Source: CAD feature listing. Evaluate the final solid. Frame: model axes, mm. Face numbers are marked on the shaded views. A direction names the side the tool comes from. Round coordinates to 2 decimals unless told otherwise and drop trailing zeros. Loops run counter-clockwise (first coordinate to the right, second up) from the corner with the lowest first, then second, coordinate; pieces in that order, holes last.
Item 1: First-contact query: P1, Ø1.8, axis at x = -1.12, z = 1.56, coming from the -Y side. Flat tip, straight axial feed; report the tip coordinate or a pass-through.
Item 2: Section query C-C on x = 0.25. Return loops of the section in (y, z), then the cut area to 3 significant figures.
Item 3: Access query for the marked faces 4, 5 and 6. Directions: +Z, -Z, +X, -X, +Y, -Y. A direction counts if a zero-diameter tool reaches every point of the face in a straight line with its end or side. Return the directions, or none.
Item 4: Section query D-D on x = 5.75. Return loops of the section in (y, z), then the cut area to 3 significant figures.
Item 5: Pull-direction query (Z, two-part tool) for the marked faces 1, 2 and 3; classes: released by +Z, released by -Z, zero draft, split by the parting line, or undercut.
Item 6: Ray query, L1, parallel to X at y = 1.2, z = 1.5; L2, parallel to Z at x = -1.5, y = 1.25; L3, parallel to X at y = 1.75, z = -4.5. Return the intervals inside material, ascending.
Item 7: Section query A-A on z = 2.75. Return loops of the section in (x, y), then the cut area to 3 significant figures.
Item 8: Section query B-B on y = 1.6. Return loops of the section in (x, z).
```python
from build123d import *

# Parameters (mm, degrees)
SKETCH1_R           = 1.5
BOSS_EXTRUDE1_DEPTH = 2


with BuildPart() as part:
    # Sketch1 → Boss-Extrude1 (new body)
    with BuildSketch(Plane(origin=(0, 0, 0), x_dir=(1, 0, 0), z_dir=(0, 1, 0))):
        with BuildLine():
            Line((6.37772525, 5.938862625), (-2.62227475, 5.938862625))
            Line((-2.62227475, 5.938862625), (-2.62227475, 3.938862625))
            Line((-2.62227475, 3.938862625), (-4.62227475, 3.938862625))
            Line((-4.62227475, 3.938862625), (-4.62227475, -2.061137375))
            ThreePointArc((-4.62227475, -2.061137375), (-3.743595093, -4.182457719), (-1.62227475, -5.061137375))
            Line((-1.62227475, -5.061137375), (4.37772525, -5.061137375))
            Line((4.37772525, -5.061137375), (4.37772525, -3.061137375))
            Line((4.37772525, -3.061137375), (6.37772525, -3.061137375))
            Line((6.37772525, -3.061137375), (6.37772525, 5.938862625))
        make_face()
        with Locations((-1.12227475, -1.561137375)):
            Circle(SKETCH1_R, mode=Mode.SUBTRACT)
    extrude(amount=BOSS_EXTRUDE1_DEPTH)


solid = part.part
```
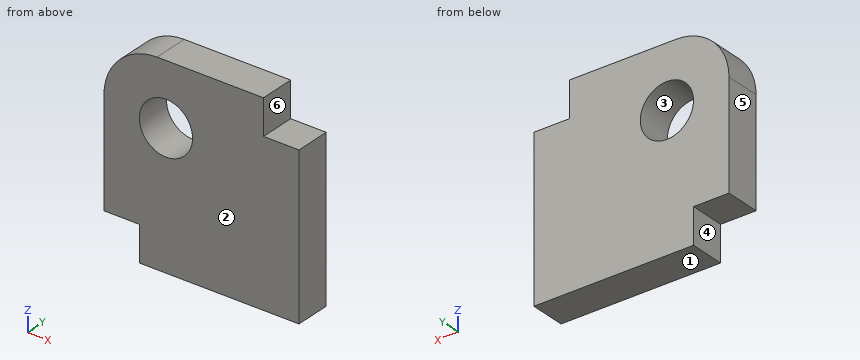
Data:
1. P1: passes through
2. outline: (0, -5.94) - (2, -5.94) - (2, 0.96) - (0, 0.96) - close; (0, 2.17) - (2, 2.17) - (2, 5.06) - (0, 5.06) - close
2. area: 19.6 mm2
3. face 4: -Z, -X, +Y, -Y
3. face 5: +Z, -Z, -X, +Y, -Y
3. face 6: +Z, +X, +Y, -Y
4. outline: (0, -5.94) - (2, -5.94) - (2, 3.06) - (0, 3.06) - close
4. area: 18.0 mm2
5. face 1: released by -Z
5. face 2: zero draft
5. face 3: undercut
6. L1: x = -4.62 to -2.62, 0.38 to 6.38
6. L2: z = -5.94 to 0.11, 3.01 to 5.06
6. L3: x = -2.62 to 6.38
7. outline: (-4.54, 0) - (-2.04, 0) - (-2.04, 2) - (-4.54, 2) - close; (-0.21, 0) - (6.38, 0) - (6.38, 2) - (-0.21, 2) - close
7. area: 18.2 mm2
8. outline: (-4.62, -3.94) - (-2.62, -3.94) - (-2.62, -5.94) - (6.38, -5.94) - (6.38, 3.06) - (4.38, 3.06) - (4.38, 5.06) - (-1.62, 5.06) arc R3 ccw to (-4.62, 2.06) - close; hole circle Ø3 at (-1.12, 1.56)
